from build123d import *

# Parameters (mm, degrees)
F0_W     = 177.8
F0_H     = 76.2
F5_DEPTH = 156.920815
F1_R     = 45.202558
F2_DEPTH = 72.338598
F3_R     = 10.618038
F3_R_2   = 11.724793
F4_DEPTH = 25.4


with BuildPart() as f5:
    # F0 (on Front) → F5 (new body)
    with BuildSketch(Plane.XZ):
        with Locations((67.268712, 38.1)):
            Rectangle(F0_W, F0_H)
    extrude(amount=F5_DEPTH)

    # F1 (on face) → F2 (cut)
    with BuildSketch(Plane.XY.offset(76.2)):
        with Locations((88.101327, -90.911075)):
            Circle(F1_R)
    extrude(amount=-F2_DEPTH, mode=Mode.SUBTRACT)

    # F3 (on face) → F4 (cut)
    with BuildSketch(Plane.XZ.offset(156.920815)):
        with Locations((13.535074, 54.284833)):
            Circle(F3_R)
        with Locations((126.181513, 20.620376)):
            Circle(F3_R_2)
    extrude(amount=-F4_DEPTH, mode=Mode.SUBTRACT)


solid = f5.part
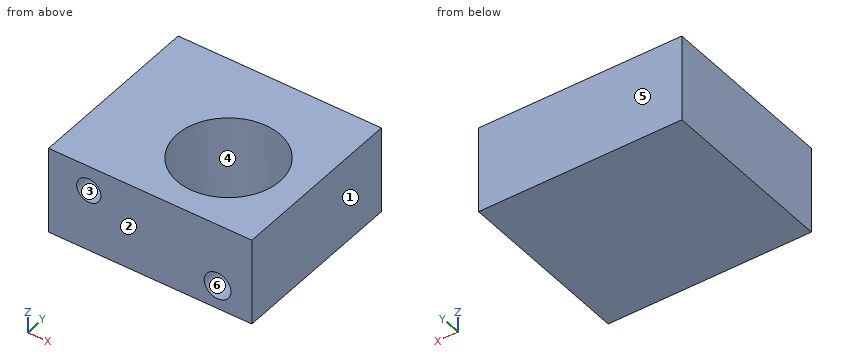
Build history of the part. All positions in model axes, mm. Face numbers are marked on the shaded views. A direction names the side the tool comes from. Give positions to 0.01 mm unless a question says otherwise; leave off trailing zeros. Loops run counter-clockwise (first coordinate to the right, second up) from the corner with the lowest first, then second, coordinate; pieces in that order, holes last. Notation, with made-up numbers: (26, 84.5) -> (59, 84.5) arc R16 cw to (59, 99.5) -> close; hole circle Ø1 at (86, 9). An arc over 180 degrees is marked (long way). Answer in a Markdown table with one row per item.
Item 1: Slice it at C-C on y = -62. Write the cut outline in (x, z).
Findings below:
| item | result |
|---|---|
| outline | (-21.63, 0) -> (156.17, 0) -> (156.17, 76.2) -> (122.85, 76.2) -> (122.85, 3.86) -> (53.35, 3.86) -> (53.35, 76.2) -> (-21.63, 76.2) -> close |
Item 2: Slice it at A-A on x = 59. Write the cut outline in (y, z), plus the area to 3 significant figures.
Findings below:
| item | result |
|---|---|
| outline | (-156.92, 0) -> (0, 0) -> (0, 76.2) -> (-56.32, 76.2) -> (-56.32, 3.86) -> (-125.5, 3.86) -> (-125.5, 76.2) -> (-156.92, 76.2) -> close |
| area | 6,950 mm² |
Item 3: Tool access for the marked faces 5 and 6: list every direction of +Z, -Z, +X, -X, +Y, -Y with a clear straight run to the whole face (end or side of a thin tool).
Findings below:
| item | result |
|---|---|
| face 5 | +Z, -Z, +X, -X, +Y |
| face 6 | -Y |
Item 4: Slice it at D-D on z = 62. Write the cut outline in (x, y), plus the area to 3 significant figures.
Findings below:
| item | result |
|---|---|
| outline | (-21.63, -156.92) -> (6.24, -156.92) -> (6.24, -131.52) -> (20.83, -131.52) -> (20.83, -156.92) -> (156.17, -156.92) -> (156.17, 0) -> (-21.63, 0) -> close; hole circle Ø90.41 at (88.1, -90.91) |
| area | 21,100 mm² |
Item 5: Mould opens along X. For the marked faces 1, 2, 3 and 4 say: pulls with the +X half, pulls with the -X half, needs draft (parallel to the pull), parting line crosses it, or undercut.
Findings below:
| item | result |
|---|---|
| face 1 | pulls with the +X half |
| face 2 | needs draft |
| face 3 | undercut |
| face 4 | undercut |
Item 6: Slice it at B-B on z = 41. Write the cut outline in (x, y), plus the area to 3 significant figures.
Findings below:
| item | result |
|---|---|
| outline | (-21.63, -156.92) -> (156.17, -156.92) -> (156.17, 0) -> (-21.63, 0) -> close; hole circle Ø90.41 at (88.1, -90.91) |
| area | 21,500 mm² |
Item 7: Flat gauge pins, fed straight in: P1, Ø2, axis at x = 101.5, y = -136.5, coming from the -Z side; P2, Ø10.5, axis at x = 13.5, z = 55, coming from the -Y side. Where does each tip first touch, or does it go through?
Findings below:
| item | result |
|---|---|
| P1 | stops at z = 0 |
| P2 | stops at y = -131.52 |
Item 8: Probe line 1 along X through (y, z) = (-49.5, 9); line 2 along Z through (x, y) = (66.5, -96.5); line 3 along X through (y, z) = (-79.5, 50.5). List the from-to ranges inside material, lowest first. Write a range as [from, to].
Findings below:
| item | result |
|---|---|
| line 1 | x = [-21.63, 69.98], [106.22, 156.17] |
| line 2 | z = [0, 3.86] |
| line 3 | x = [-21.63, 44.36], [131.84, 156.17] |
